from build123d import *

# Parameters (mm, degrees)
SKETCH1_W           = 45
SKETCH1_H           = 5
BOSS_EXTRUDE1_DEPTH = 102.5
SKETCH2_R           = 2.575
CUT_EXTRUDE1_DEPTH  = 106.059506947
SKETCH3_W           = 10
SKETCH3_H           = 1
CUT_EXTRUDE2_DEPTH  = 112.970978383
SKETCH4_W           = 45
SKETCH4_H           = 5
BOSS_EXTRUDE2_DEPTH = 35
BOSS_EXTRUDE3_DEPTH = 22.5
SKETCH6_R           = 2.575
CUT_EXTRUDE3_DEPTH  = 145.762736918
SKETCH7_R           = 2.575
CUT_EXTRUDE4_DEPTH  = 145.762736918
CUT_EXTRUDE5_DEPTH  = 145.762736918


with BuildPart() as part:
    # Sketch1 → Boss-Extrude1 (new body)
    with BuildSketch(Plane.XY):
        Rectangle(SKETCH1_W, SKETCH1_H)
    boss_extrude1 = extrude(amount=BOSS_EXTRUDE1_DEPTH)

    # Sketch2 → Cut-Extrude1 (cut, through all)
    with BuildSketch(Plane(origin=(0, 2.5, 0), x_dir=(1, 0, 0), z_dir=(0, 1, 0))):
        with Locations(Location((-15, -59, 0), (0, 0, 270))):
            Circle(SKETCH2_R)
        with Locations(Location((15, -59, 0), (0, 0, 270))):
            Circle(SKETCH2_R)
        with Locations(Location((-15, -91, 0), (0, 0, 270))):
            Circle(SKETCH2_R)
        with Locations(Location((15, -91, 0), (0, 0, 270))):
            Circle(SKETCH2_R)
    cut_extrude1 = extrude(amount=-CUT_EXTRUDE1_DEPTH, mode=Mode.SUBTRACT)

    # Sketch3 → Cut-Extrude2 (cut, through all)
    with BuildSketch(Plane(origin=(22.5, 0, 0), x_dir=(0, 0, -1), z_dir=(1, 0, 0))):
        with Locations((-75, 2)):
            Rectangle(SKETCH3_W, SKETCH3_H)
    cut_extrude2 = extrude(amount=-CUT_EXTRUDE2_DEPTH, mode=Mode.SUBTRACT)

    # Mirror1: Boss-Extrude1, Cut-Extrude1, Cut-Extrude2 across plane
    add(boss_extrude1.mirror(Plane.XY))
    add(cut_extrude1.mirror(Plane.XY), mode=Mode.SUBTRACT)
    add(cut_extrude2.mirror(Plane.XY), mode=Mode.SUBTRACT)

    # Sketch4 → Boss-Extrude2 (add)
    with BuildSketch(Plane.XY.offset(102.5)):
        Rectangle(SKETCH4_W, SKETCH4_H)
    extrude(amount=BOSS_EXTRUDE2_DEPTH)

    # Sketch5 → Boss-Extrude3 (add)
    with BuildSketch(Plane(origin=(22.5, 0, 0), x_dir=(0, 0, -1), z_dir=(1, 0, 0))):
        Polygon((70, 1.5), (70, 2.5), (-70, 2.5), (-70, 1.5), (-80, 1.5), (-80, 2.5), (-137.5, 2.5), (-137.5, -2.5), (102.5, -2.5), (102.5, 2.5), (80, 2.5), (80, 1.5), align=None)
    boss_extrude3 = extrude(amount=BOSS_EXTRUDE3_DEPTH)

    # Mirror2: Boss-Extrude3 across plane
    add(boss_extrude3.mirror(Plane(origin=(0, 0, 0), x_dir=(0, 0, 1), z_dir=(1, 0, 0))))

    # Sketch6 → Cut-Extrude3 (cut, through all)
    with BuildSketch(Plane(origin=(0, 2.5, 0), x_dir=(1, 0, 0), z_dir=(0, 1, 0))):
        with Locations(Location((-35, -17.5, 0), (0, 0, 270))):
            Circle(SKETCH6_R)
        with Locations(Location((-35, 17.5, 0), (0, 0, 270))):
            Circle(SKETCH6_R)
    cut_extrude3 = extrude(amount=-CUT_EXTRUDE3_DEPTH, mode=Mode.SUBTRACT)

    # Mirror3: Cut-Extrude3 across plane
    add(cut_extrude3.mirror(Plane(origin=(0, 0, 0), x_dir=(0, 0, 1), z_dir=(1, 0, 0))), mode=Mode.SUBTRACT)

    # Sketch7 → Cut-Extrude4 (cut, through all)
    with BuildSketch(Plane(origin=(0, 2.5, 0), x_dir=(1, 0, 0), z_dir=(0, 1, 0))):
        with Locations(Location((-25, -126.5, 0), (0, 0, 270))):
            Circle(SKETCH7_R)
        with Locations(Location((25, -126.5, 0), (0, 0, 90))):
            Circle(SKETCH7_R)
    extrude(amount=-CUT_EXTRUDE4_DEPTH, mode=Mode.SUBTRACT)

    # Sketch8 → Cut-Extrude5 (cut, through all)
    with BuildSketch(Plane(origin=(0, 2.5, 0), x_dir=(1, 0, 0), z_dir=(0, 1, 0))):
        with BuildLine():
            Line((-17.575, -111.5), (-17.575, -102.5))
            ThreePointArc((-17.575, -102.5), (-15, -99.925), (-12.425, -102.5))
            Line((-12.425, -102.5), (-12.425, -111.5))
            ThreePointArc((-12.425, -111.5), (-15, -114.075), (-17.575, -111.5))
        make_face()
        with BuildLine():
            Line((17.575, -111.5), (17.575, -102.5))
            ThreePointArc((17.575, -102.5), (15, -99.925), (12.425, -102.5))
            Line((12.425, -102.5), (12.425, -111.5))
            ThreePointArc((12.425, -111.5), (15, -114.075), (17.575, -111.5))
        make_face()
    extrude(amount=-CUT_EXTRUDE5_DEPTH, mode=Mode.SUBTRACT)


solid = part.part
Verification items for the finished model (mm, model axes). A direction names the side the tool comes from. Give positions to 0.01 mm unless a question says otherwise; leave off trailing zeros. Write each loop counter-clockwise with the first axis right and the second up, starting at its lowest first coordinate (ties: lowest second). Pieces come first, ordered by that corner, then holes.
(1) Cross-section at A-A (z = -17.5). Enter the section's corners in (x, y) (3 decimals), plus the area to 4 significant figures.
(2) Material ranges on line 1 (Z direction, x = 6, y = 1.6); line 2 (X direction, y = -1.4, z = -17.5) (3 decimals); line 3 (Z direction, x = 24.5, y = 1.65), recorded low to high.
(3) Cross-section at B-B (x = -15). State how many separate pieces and enclosed holes the cut face has, plus the area to 3 significant figures.
(4) Cross-section at C-C (x = 35). Enter the section's corners in (y, z) (3 decimals), plus the area to 3 significant figures.
(5) Access from +Z, -Z, +X, -X, +Y, -Y to the whole of each face (thin tool, end or side, straight path). Record for faces 4 (the face through (-17.575, 0, 107)), 5 (the face through (1, -2.5, 19)).
(6) Mould release check, pull along X, two halves, no side actions. Record for faces 1 (the face through (-45, 0, 19)), 2 (the face through (1, 0, 137.5)), 3 (the face through (-17.284, 0.035, -92.188)): +X half, -X half, draft (parallel to the pull), parting line (faces both ways), or undercut.
(7) Gauge pin test, flat end, axial feed: pin 1 (4 mm diameter, centred on x = -35, z = 17.5, fed in from -Y). Record the tip position at first contact, or that the pin passes through.
Worked out:
1. outline: (-45, -2.5) - (-37.575, -2.5) - (-37.575, 2.5) - (-45, 2.5) - close; (-32.425, -2.5) - (32.425, -2.5) - (32.425, 2.5) - (-32.425, 2.5) - close; (37.575, -2.5) - (45, -2.5) - (45, 2.5) - (37.575, 2.5) - close
1. area: 398.5 mm2
2. line 1: z = -102.5 to -80, -70 to 70, 80 to 137.5
2. line 2: x = -45 to -37.575, -32.425 to 32.425, 37.575 to 45
2. line 3: z = -102.5 to -80, -70 to 70, 80 to 123.97, 129.03 to 137.5
3. separate pieces: 6
3. enclosed holes: 0
3. area: 1,010 mm2
4. outline: (-2.5, -102.5) - (2.5, -102.5) - (2.5, -80) - (1.5, -80) - (1.5, -70) - (2.5, -70) - (2.5, -20.075) - (-2.5, -20.075) - close; (-2.5, -14.925) - (2.5, -14.925) - (2.5, 14.925) - (-2.5, 14.925) - close; (-2.5, 20.075) - (2.5, 20.075) - (2.5, 70) - (1.5, 70) - (1.5, 80) - (2.5, 80) - (2.5, 137.5) - (-2.5, 137.5) - close
4. area: 1,130 mm2
5. face 4: +Y, -Y
5. face 5: +Z, -Z, +X, -X, -Y
6. face 1: -X half
6. face 2: draft
6. face 3: undercut
7. pin 1: passes through
